Read the model definition and answer for the solid it produces. Units are mm, in the model's axes. Face numbers are marked on the shaded views. A direction names the side the tool comes from. Coordinates: 2 decimals unless noted, no trailing zeros. Write each loop counter-clockwise with the first axis right and the second up, starting at its lowest first coordinate (ties: lowest second). Pieces come first, ordered by that corner, then holes.
(1) Given pin 1 (4 mm diameter, centred on x = -22, z = 9, fed in from -Y); pin 2 (6.5 mm diameter, centred on y = -3.16, z = 0, fed in from +X) (3 decimals); pin 3 (1 mm diameter, centred on x = -21, y = -19, fed in from +Z); pin 4 (6.5 mm diameter, centred on x = 38, z = 0, fed in from -Y), each flat-ended and moving along its own axis, determine where each tip first touches the part or whether it passes through.
(2) Section D-D on z = -113 is taken. Write down the section's boundary in (x, y) (1 decimal), then the cut area to 3 significant figures.
(3) Find the intervals of material crossed by probe 1 along Y at (x, z) = (-5.5, -29); probe 2 along X at (y, z) = (6.8, 0) (3 decimals); probe 3 along X at (y, z) = (-9.75, -19.05) (3 decimals), in increasing order.
(4) Section C-C on y = -33 is taken. Write down the section's boundary in (x, z) (1 decimal), then the cut area to 3 significant figures.
(5) Which of the six approach directions +Z, -Z, +X, -X, +Y, -Y give full straight-line access (tool end or side, diameter ignored) to the marked faces 1, 2 and 3?
(6) Section A-A on x = 0 is taken. State how many separate pieces and enclosed holes the cut face has, then the cut area to 3 significant figures.
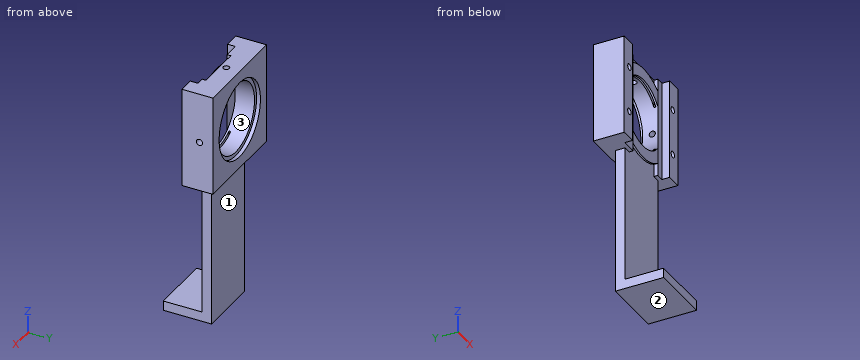
from build123d import *

# Parameters (mm, degrees)
BOSS_EXTRUDE1_DEPTH          = 7.9375
SKETCH2_W                    = 50.8
SKETCH2_H                    = 7.9375
BOSS_EXTRUDE2_DEPTH          = 31.75
SKETCH8_W                    = 82.55
SKETCH8_H                    = 82.55
BOSS_EXTRUDE6_DEPTH          = 7.9375
SKETCH10_R                   = 6.35
CENTER_HOLE_DEPTH            = 15.875
SKETCH12_W                   = 12.7
SKETCH12_H                   = 82.55
CLAMP_PAD_DEPTH              = 9.525
SKETCH13_W                   = 12.7
SKETCH13_H                   = 82.55
SKETCH13_W_2                 = 6.35
WEAR_PAD_DEPTH               = 3.175
SKETCH14_W                   = 82.55
SKETCH14_H                   = 82.55
BOSS_EXTRUDE10_DEPTH         = 0.014283
SKETCH15_R                   = 28.575
CUT_EXTRUDE3_DEPTH           = 19.05
BOSS_EXTRUDE7_START          = 1.5875
SKETCH11_R                   = 38.1
SKETCH11_R_2                 = 28.575
BOSS_EXTRUDE7_DEPTH          = 1.5875
SKETCH24_R                   = 31.75
CUT_EXTRUDE4_DEPTH           = 3.175
F_1_4_20_TAPPED_HOLE5_REACH  = 213.114
F_1_4_20_TAPPED_HOLE5_BORE_R = 2.5527
F_1_4_20_TAPPED_HOLE6_REACH  = 188.036
F_1_4_20_TAPPED_HOLE6_BORE_R = 2.5527
F_1_4_20_TAPPED_HOLE7_D      = 5.1054
F_1_4_20_TAPPED_HOLE7_DEPTH  = 16.51
F_1_4_20_TAPPED_HOLE7_TIP    = 1.533816902
F_1_4_20_TAPPED_HOLE8_D      = 5.1054
F_1_4_20_TAPPED_HOLE8_DEPTH  = 16.51
F_1_4_20_TAPPED_HOLE8_TIP    = 1.533816902


with BuildPart() as part:
    # Sketch1 → Boss-Extrude1 (new body)
    with BuildSketch(Plane(origin=(0, 0, 0), x_dir=(1, 0, 0), z_dir=(0, 1, 0))):
        Polygon((-22.225, 41.275), (-41.275, 41.275), (-41.275, -41.275), (41.275, -41.275), (41.275, 41.275), (28.575, 41.275), (28.575, 161.925), (-22.225, 161.925), align=None)
    extrude(amount=-BOSS_EXTRUDE1_DEPTH)

    # Sketch2 → Boss-Extrude2 (add)
    with BuildSketch(Plane.XZ.offset(7.9375)):
        with Locations((3.175, -157.95625)):
            Rectangle(SKETCH2_W, SKETCH2_H)
    extrude(amount=BOSS_EXTRUDE2_DEPTH)

    # Sketch8 → Boss-Extrude6 (add)
    with BuildSketch(Plane(origin=(0, 0, 0), x_dir=(1, 0, 0), z_dir=(0, 1, 0))):
        Rectangle(SKETCH8_W, SKETCH8_H)
    extrude(amount=BOSS_EXTRUDE6_DEPTH)

    # Sketch10 → Center Hole (cut)
    with BuildSketch(Plane(origin=(0, 7.9375, 0), x_dir=(1, 0, 0), z_dir=(0, 1, 0))):
        with Locations(Location((0, 0, 0), (0, 0, 270))):
            Circle(SKETCH10_R)
    extrude(amount=-CENTER_HOLE_DEPTH, mode=Mode.SUBTRACT)

    # Sketch12 → Clamp Pad (add)
    with BuildSketch(Plane.XZ.offset(7.9375)):
        with Locations((-34.925, 0)):
            Rectangle(SKETCH12_W, SKETCH12_H)
        with Locations((34.925, 0)):
            Rectangle(SKETCH12_W, SKETCH12_H)
    extrude(amount=CLAMP_PAD_DEPTH)

    # Sketch13 → Wear Pad (add)
    with BuildSketch(Plane.XZ.offset(7.9375)):
        with Locations((-22.225, 0)):
            Rectangle(SKETCH13_W, SKETCH13_H)
        with Locations((25.4, 0)):
            Rectangle(SKETCH13_W_2, SKETCH13_H)
    extrude(amount=WEAR_PAD_DEPTH)

    # Sketch14 → Boss-Extrude10 (add)
    with BuildSketch(Plane(origin=(0, 7.9375, 0), x_dir=(1, 0, 0), z_dir=(0, 1, 0))):
        Rectangle(SKETCH14_W, SKETCH14_H)
    extrude(amount=BOSS_EXTRUDE10_DEPTH)

    # Sketch15 → Cut-Extrude3 (cut)
    with BuildSketch(Plane(origin=(0, 7.951783292, 0), x_dir=(1, 0, 0), z_dir=(0, 1, 0))):
        with Locations(Location((0, 0, 0), (0, 0, 270))):
            Circle(SKETCH15_R)
    extrude(amount=-CUT_EXTRUDE3_DEPTH, mode=Mode.SUBTRACT)

    # Sketch11 → Boss-Extrude7 (add)
    with BuildSketch(Plane(origin=(0, -11.098216708, 0), x_dir=(1, 0, 0), z_dir=(0, 1, 0)).offset(BOSS_EXTRUDE7_START)):
        Circle(SKETCH11_R)
        with Locations(Location((0, 0, 0), (0, 0, 270))):
            Circle(SKETCH11_R_2, mode=Mode.SUBTRACT)
    extrude(amount=-BOSS_EXTRUDE7_DEPTH)

    # Sketch24 → Cut-Extrude4 (cut)
    with BuildSketch(Plane(origin=(0, 7.951783292, 0), x_dir=(1, 0, 0), z_dir=(0, 1, 0))):
        with Locations(Location((0, 0, 0), (0, 0, 270))):
            Circle(SKETCH24_R)
    extrude(amount=-CUT_EXTRUDE4_DEPTH, mode=Mode.SUBTRACT)

    # 1/4-20 Tapped Hole5 bore → 1/4-20 Tapped Hole5 (cut, up to next)
    with BuildSketch(Plane.XY.offset(41.275), mode=Mode.PRIVATE) as f_1_4_20_tapped_hole5_sk1:
        with Locations((0, -3.160716708)):
            Circle(F_1_4_20_TAPPED_HOLE5_BORE_R)
    f_1_4_20_tapped_hole5_tool1 = extrude(f_1_4_20_tapped_hole5_sk1.sketch, amount=-F_1_4_20_TAPPED_HOLE5_REACH, mode=Mode.PRIVATE) & part.part
    add(f_1_4_20_tapped_hole5_tool1.solids().sort_by_distance((0, -3.160717, 41.275))[0], mode=Mode.SUBTRACT)

    # 1/4-20 Tapped Hole6 bore → 1/4-20 Tapped Hole6 (cut, up to next)
    with BuildSketch(Plane(origin=(41.275, 0, 0), x_dir=(0, 0, -1), z_dir=(1, 0, 0)), mode=Mode.PRIVATE) as f_1_4_20_tapped_hole6_sk1:
        with Locations((0, -3.160716708)):
            Circle(F_1_4_20_TAPPED_HOLE6_BORE_R)
    f_1_4_20_tapped_hole6_tool1 = extrude(f_1_4_20_tapped_hole6_sk1.sketch, amount=-F_1_4_20_TAPPED_HOLE6_REACH, mode=Mode.PRIVATE) & part.part
    add(f_1_4_20_tapped_hole6_tool1.solids().sort_by_distance((41.275, -3.160717, 0))[0], mode=Mode.SUBTRACT)

    # 1/4-20 Tapped Hole7
    with Locations(Plane(origin=(0, -17.4625, 0), x_dir=(-1, 0, 0), z_dir=(0, -1, 0))):
        with Locations((33.3375, 19.05), (33.3375, -19.05)):
            Hole(F_1_4_20_TAPPED_HOLE7_D / 2, depth=F_1_4_20_TAPPED_HOLE7_DEPTH)
            with Locations((0, 0, -(F_1_4_20_TAPPED_HOLE7_DEPTH + F_1_4_20_TAPPED_HOLE7_TIP / 2))):  # 118° drill point
                Cone(0, F_1_4_20_TAPPED_HOLE7_D / 2, F_1_4_20_TAPPED_HOLE7_TIP, mode=Mode.SUBTRACT)

    # 1/4-20 Tapped Hole8
    with Locations(Plane(origin=(0, -17.4625, 0), x_dir=(-1, 0, 0), z_dir=(0, -1, 0))):
        with Locations((-33.3375, 19.05), (-33.3375, -19.05)):
            Hole(F_1_4_20_TAPPED_HOLE8_D / 2, depth=F_1_4_20_TAPPED_HOLE8_DEPTH)
            with Locations((0, 0, -(F_1_4_20_TAPPED_HOLE8_DEPTH + F_1_4_20_TAPPED_HOLE8_TIP / 2))):  # 118° drill point
                Cone(0, F_1_4_20_TAPPED_HOLE8_D / 2, F_1_4_20_TAPPED_HOLE8_TIP, mode=Mode.SUBTRACT)


solid = part.part
Response:
1. pin 1: stops at y = -11.11
1. pin 2: stops at x = 41.275
1. pin 3: stops at z = -153.99
1. pin 4: stops at y = -17.46
2. outline: (-22.2, -7.9) - (28.6, -7.9) - (28.6, 0) - (-22.2, 0) - close
2. area: 403 mm2
3. probe 1: y = -11.1 to -9.51, -7.94 to 4.78
3. probe 2: x = -41.275 to -31.75, 31.75 to 41.275
3. probe 3: x = -41.275 to -35.89, -30.785 to -21.299, 21.299 to 30.785, 35.89 to 41.275
4. outline: (-22.2, -161.9) - (28.6, -161.9) - (28.6, -154) - (-22.2, -154) - close
4. area: 403 mm2
5. face 1: -Z, +X, -X, +Y
5. face 2: -Z, +X, -X, +Y, -Y
5. face 3: +Y
6. separate pieces: 5
6. enclosed holes: 0
6. area: 1,560 mm2
